```python
from build123d import *

# Parameters (mm, degrees)
F1_DEPTH = 12.7


with BuildPart() as f1:
    # F0 (on Front) → F1 (new body, symmetric)
    with BuildSketch(Plane.XZ):
        with BuildLine():
            Line((-19.05, -52.705), (19.05, -52.705))
            Line((19.05, -52.705), (19.05, -63.275363))
            Line((19.05, -63.275363), (34.081931, -72.595161))
            Line((34.081931, -72.595161), (34.081931, -62.168677))
            Line((34.081931, -62.168677), (19.05, -39.198428))
            Line((19.05, -39.198428), (19.05, -31.643265))
            Line((19.05, -31.643265), (75.1586, -39.198428))
            Line((75.1586, -39.198428), (75.1586, -18.334107))
            Line((75.1586, -18.334107), (19.05, 23.027632))
            Line((19.05, 23.027632), (19.05, 52.705))
            Line((19.05, 52.705), (11.364806, 52.705))
            Line((11.364806, 52.705), (11.364806, 67.008361))
            ThreePointArc((11.364806, 67.008361), (8.475728, 89.264488), (0, 110.045344))
            ThreePointArc((0, 110.045344), (-6.504109, 88.962248), (-8.701194, 67.008361))
            Line((-8.701194, 67.008361), (-8.701194, 52.705))
            Line((-8.701194, 52.705), (-19.05, 52.705))
            Line((-19.05, 52.705), (-19.05, 23.027632))
            Line((-19.05, 23.027632), (-75.1586, -18.334107))
            Line((-75.1586, -18.334107), (-75.1586, -39.198428))
            Line((-75.1586, -39.198428), (-23.7749, -30.977035))
            Line((-23.7749, -30.977035), (-19.05, -30.977035))
            Line((-19.05, -30.977035), (-19.05, -39.198428))
            Line((-19.05, -39.198428), (-34.611922, -62.3945))
            Line((-34.611922, -62.3945), (-34.611922, -72.377621))
            Line((-34.611922, -72.377621), (-19.181741, -63.053779))
            Line((-19.181741, -63.053779), (-19.05, -52.705))
        make_face()
        Polygon((19.05, -30.977035), (19.05, -31.643265), (14.102228, -30.977035), align=None, mode=Mode.SUBTRACT)
        Polygon((14.102228, -30.977035), (19.05, -31.643265), (19.05, -30.977035), align=None)
    extrude(amount=F1_DEPTH, both=True)


solid = f1.part
```
Geometry: final body of the model. Coordinates: model frame, mm. A direction names the side the tool comes from. Give positions to 0.01 mm unless a question says otherwise; leave off trailing zeros. Write each loop counter-clockwise with the first axis right and the second up, starting at its lowest first coordinate (ties: lowest second). Pieces come first, ordered by that corner, then holes.
1. Line query: probe 1 along X at (y, z) = (-10.75, 45); probe 2 along X at (y, z) = (-0.25, -54); probe 3 along Z at (x, y) = (-15.5, -8.75) (3 decimals). Output: solid intervals per line, ascending.
2. Reachability of faces 4 (the flat face through (26.67, -0.18, -50.84)), 5 (the flat face through (34.082, 0, -67)), 6 (the flat face through (-14, 0, 52.705)) from +Z, -Z, +X, -X, +Y, -Y: full face, straight path, thin tool, end or side. Return the list, or none.
3. Draft query along Z for faces 1 (the cylindrical face through (-6.44, -0.18, 89.27)), 2 (the flat face through (46.712, -0.178, -35.368)), 3 (the flat face through (-19.05, 0, 38)). Return one class per face: released by +Z, released by -Z, zero draft, split by the parting line, or undercut.
4. Section query C-C, the plane z = 63. Return loops of the section in (x, y), then the cut area to 3 significant figures.
5. Pin query (flat end, axial travel): P1, Ø1.5, axis at y = 8, z = 28, coming from the -X side; P2, Ø3, axis at x = -15, y = 3, coming from the +Z side (3 decimals); P3, Ø2.5, axis at x = -22.5, y = 6, coming from the -Z side. Return the tip coordinate at first contact, or that it passes through.
6. Section query D-D, the plane x = 49. Return loops of the section in (y, z), then the cut area to 3 significant figures.
7. Section query A-A, the plane x = -28. Return loops of the section in (y, z).
Computed:
1. probe 1: x = -19.05 to 19.05
1. probe 2: x = -28.98 to -19.07, 19.05 to 28.74
1. probe 3: z = -52.705 to 52.705
2. face 4: +X, +Y, -Y
2. face 5: -Z, +X, +Y, -Y
2. face 6: +Z, -X, +Y, -Y
3. face 1: released by +Z
3. face 2: undercut
3. face 3: zero draft
4. outline: (-8.7, -12.7) - (11.36, -12.7) - (11.36, 12.7) - (-8.7, 12.7) - close
4. area: 510 mm2
5. P1: stops at x = -19.05
5. P2: stops at z = 52.705
5. P3: stops at z = -65.81
6. outline: (-12.7, -35.68) - (12.7, -35.68) - (12.7, 0.95) - (-12.7, 0.95) - close
6. area: 930 mm2
7. outline: (-12.7, -68.38) - (12.7, -68.38) - (12.7, -52.54) - (-12.7, -52.54) - close; (-12.7, -31.65) - (12.7, -31.65) - (12.7, 16.43) - (-12.7, 16.43) - close
